Model file for the job. Use its own axes, mm. Give positions to 0.01 mm unless a question says otherwise; leave off trailing zeros. Loops run counter-clockwise (first coordinate to the right, second up) from the corner with the lowest first, then second, coordinate; pieces in that order, holes last. Notation, with made-up numbers: M -4.5,14.25 L 15.5,14.25 A21 cw 15.5,18.25 Z; hole C -1.5,-20 d9. An arc over 180 degrees is marked long. Answer in a Markdown table with one row per item.
```python
from build123d import *

# Parameters (mm, degrees)
F0_R            = 300
F1_DEPTH        = 25
F3_DEPTH        = 25
F3_COPIES_COUNT = 18


# Not quite as in the source:
# - a pattern or mirror of a feature is missing from the dataset's text; its kind, count and spacing are read off the source's solid


with BuildPart() as f1:
    # F0 (on Front) → F1 (new body)
    with BuildSketch(Plane.XZ):
        Circle(F0_R)
    extrude(amount=F1_DEPTH)

    # F2 (on face) → F3 (join, through all)
    with BuildSketch(Plane.XZ.offset(25)):
        with BuildLine():
            ThreePointArc((43.9549568499, 296.7624669131), (46.962798618, 296.1906436564), (50, 295.803989155))
            ThreePointArc((50, 295.803989155), (46.9799228296, 296.2986446998), (43.9549568499, 296.7624669131))
        make_face()
        with BuildLine():
            ThreePointArc((-50, 295.803989155), (-46.962798618, 296.1906436564), (-43.9549568499, 296.7624669131))
            ThreePointArc((-43.9549568499, 296.7624669131), (-46.9799228296, 296.2986446998), (-50, 295.803989155))
        make_face()
        with BuildLine():
            ThreePointArc((-43.9549568499, 296.7624669131), (0, 300), (43.9549568499, 296.7624669131))
            ThreePointArc((43.9549568499, 296.7624669131), (17.1882851118, 312.6207310432), (4.9811623415, 341.2376038778))
            ThreePointArc((4.9811623415, 341.2376038778), (0, 345.803989155), (-4.9811623415, 341.2376038778))
            ThreePointArc((-4.9811623415, 341.2376038778), (-17.1882851118, 312.6207310432), (-43.9549568499, 296.7624669131))
        make_face()
    f3 = extrude(amount=-F3_DEPTH)

    # F3_copies: F3 ×18 about axis
    f3_copies_axis = Axis((0, 0, 0), (0, 1, 0))
    for i in range(1, F3_COPIES_COUNT):
        add(f3.rotate(f3_copies_axis, i * 360 / F3_COPIES_COUNT))


solid = f1.part
```
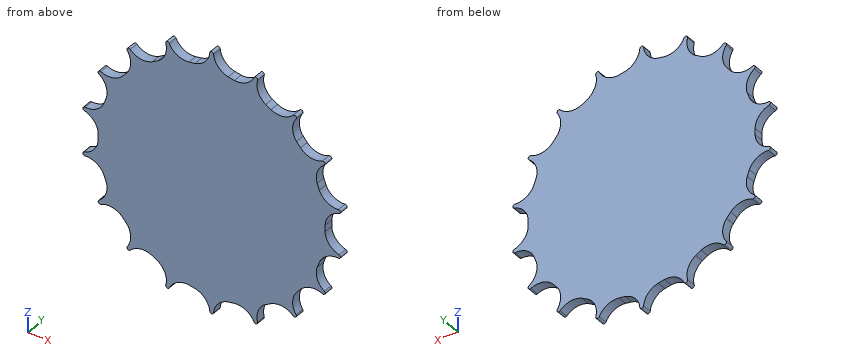
Q1. Probe probe 1 along X at (y, z) = (-15.5, -255); probe 2 along Z at (x, y) = (286, -17.75); probe 3 along Z at (x, y) = (66.5, -13.25). List the from-to ranges inside material, lowest first.
Reported:
| item | result |
|---|---|
| probe 1 | -221.09 to -202.06, -158.25 to 158.25, 202.06 to 221.09 |
| probe 2 | -172.27 to -154.42, -91.78 to 91.78, 154.42 to 172.27 |
| probe 3 | -293.47 to 293.47 |
Q2. Saw through at A-A (z = 122.5). Give the cut face in (x, y).
Reported:
| item | result |
|---|---|
| outline | M -276.75,-25 L 276.75,-25 L 276.75,0 L -276.75,0 Z |
Q3. Saw through at B-B (x = -167.5). Give the cut face in (y, z).
Reported:
| item | result |
|---|---|
| outline | M -25,-251.57 L 0,-251.57 L 0,251.57 L -25,251.57 Z |
Q4. Drop flat-ended pins along their axis: pin 1 (5 mm diameter, centred on y = -20.5, z = 142.5, fed in from +X); pin 2 (4 mm diameter, centred on y = -12.5, z = 29, fed in from -X); pin 3 (12 mm diameter, centred on y = -4.5, z = 274.5, fed in from +X). Give the stop position or say it passes through.
Reported:
| item | result |
|---|---|
| pin 1 | x = 280.7 |
| pin 2 | x = -306.51 |
| pin 3 | x = 136.6 |
